Here's how the part is built. I have some questions about the finished solid (model axes, mm). A direction names the side the tool comes from. Give positions to 0.01 mm unless a question says otherwise; leave off trailing zeros. Order: outer loops, then holes, each group sorted by start corner. A loop starts at its lowest first (then second) coordinate and runs counter-clockwise, first axis right, second up. Notation, with made-up numbers: (-14.75, 74.25) -> (0.25, 74.25) arc R8 ccw to (0.25, 84.25) -> close; hole circle Ø1 at (35.5, 69.5). An arc over 180 degrees is marked (long way). Write each question's results on one line, items separated by ' | '. Start each with the question number.
Q1. Thinking about a two-plate mould opening in Y: for faces 1 (the face through (2, -12, 0)), 2 (the face through (2, 18.918, 5)), 3 (the face through (34.04, -44.075, 0.986)), which applies, pulls with the +Y half, pulls with the -Y half, needs draft (parallel to the pull), parting line crosses it, or undercut?
Q2. Imagine slicing it at A-A, the plane z = 5. Please give me the cut outline in (x, y), then the cut area to 3 significant figures.
Q3. I need wall thicknesses on line 1 along Y through (x, z) = (26.5, 5); line 2 along X through (y, z) = (-32.5, 8.5); line 3 along Z through (x, y) = (-9.5, -15). Which ranges of each line are inside material? Lowest first, please. Write a range as [from, to].
Q4. Imagine slicing it at C-C, the plane x = -18. Please give me the cut outline in (y, z), then the cut area to 3 significant figures.
Q5. For faces 4 (the face through (31.087, 17.207, 5.451)), 5 (the face through (33.91, 7.35, 5.45)), 6 (the face through (32.61, -42.676, 5.451)), which set-ups out of +Z, -Z, +X, -X, +Y, -Y let a thin tool reach every point of the face, with its end or its side?
Q6. Imagine slicing it at B-B, the plane y = 3. Please give me the cut outline in (x, z), then the cut area to 3 significant figures.
Q7. I'm going to push flat-ended pins straight in: pin 1 (2 mm diameter, centred on y = -2.5, z = 4, fed in from +X); pin 2 (6 mm diameter, centred on x = -3.5, y = -10, fed in from +Z); pin 3 (1.8 mm diameter, centred on y = 5.92, z = 5, fed in from -X). Where does each tip first touch, or does it pass through?
```python
from build123d import *

# Parameters (mm, degrees)
EXTRUDE_1_DEPTH     = 2
EXTRUDE_2_DEPTH     = 7
SHELL_1_T           = -2
SKETCH_3_R          = 1.5
CUT_EXTRUDE_1_DEPTH = 7
SKETCH_4_R          = 1.5
CUT_EXTRUDE_2_DEPTH = 7


with BuildPart() as part:
    # 草图1 → 凸台-拉伸1 (new body)
    with BuildSketch(Plane.XY):
        with BuildLine():
            Line((-23.108505897, 22.918009168), (26.891494103, 22.918009168))
            ThreePointArc((26.891494103, 22.918009168), (33.962561915, 19.989076979), (36.891494103, 12.918009168))
            Line((36.891494103, 12.918009168), (36.891494103, -37.081990832))
            ThreePointArc((36.891494103, -37.081990832), (33.962561915, -44.153058644), (26.891494103, -47.081990832))
            Line((26.891494103, -47.081990832), (-23.108505897, -47.081990832))
            ThreePointArc((-23.108505897, -47.081990832), (-30.179573709, -44.153058644), (-33.108505897, -37.081990832))
            Line((-33.108505897, -37.081990832), (-33.108505897, 12.918009168))
            ThreePointArc((-33.108505897, 12.918009168), (-30.179573709, 19.989076979), (-23.108505897, 22.918009168))
        make_face()
    extrude(amount=EXTRUDE_1_DEPTH)

    # 草图2 → 凸台-拉伸2 (add)
    with BuildSketch(Plane.XY.offset(2)):
        with BuildLine():
            Line((-23.108505897, 20.918009168), (26.891494103, 20.918009168))
            ThreePointArc((26.891494103, 20.918009168), (32.548348353, 18.574863417), (34.891494103, 12.918009168))
            Line((34.891494103, 12.918009168), (34.891494103, -37.081990832))
            ThreePointArc((34.891494103, -37.081990832), (32.548348353, -42.738845082), (26.891494103, -45.081990832))
            Line((26.891494103, -45.081990832), (-23.108505897, -45.081990832))
            ThreePointArc((-23.108505897, -45.081990832), (-28.765360146, -42.738845082), (-31.108505897, -37.081990832))
            Line((-31.108505897, -37.081990832), (-31.108505897, 12.918009168))
            ThreePointArc((-31.108505897, 12.918009168), (-28.765360146, 18.574863417), (-23.108505897, 20.918009168))
        make_face()
    extrude(amount=EXTRUDE_2_DEPTH)

    # 抽壳1
    shell_1_openings = [part.faces().sort_by_distance(p)[0] for p in [
        (1.891494103, -12.081990832, 9),
    ]]
    offset(amount=SHELL_1_T, openings=shell_1_openings, kind=Kind.INTERSECTION)

    # 草图3 → 切除-拉伸1 (cut)
    with BuildSketch(Plane.ZY.offset(31.108505897)):
        with Locations(Location((5, -30.081990832, 0), (0, 0, 270))):
            Circle(SKETCH_3_R)
    extrude(amount=-CUT_EXTRUDE_1_DEPTH, mode=Mode.SUBTRACT)

    # 草图4 → 切除-拉伸2 (cut)
    with BuildSketch(Plane(origin=(34.891494103, 0, 0), x_dir=(0, 0, -1), z_dir=(1, 0, 0))):
        with Locations(Location((-5, 5.918009168, 0), (0, 0, 90))):
            Circle(SKETCH_4_R)
    extrude(amount=-CUT_EXTRUDE_2_DEPTH, mode=Mode.SUBTRACT)


solid = part.part
```
Geometry check:
1) face 1: needs draft | face 2: undercut | face 3: pulls with the -Y half
2) outline: (-31.11, -37.08) arc R8 ccw to (-23.11, -45.08) -> (26.89, -45.08) arc R8 ccw to (34.89, -37.08) -> (34.89, 4.42) -> (32.89, 4.42) -> (32.89, -37.08) arc R6 cw to (26.89, -43.08) -> (-23.11, -43.08) arc R6 cw to (-29.11, -37.08) -> (-29.11, -31.58) -> (-31.11, -31.58) -> close; (-31.11, -28.58) -> (-29.11, -28.58) -> (-29.11, 12.92) arc R6 cw to (-23.11, 18.92) -> (26.89, 18.92) arc R6 cw to (32.89, 12.92) -> (32.89, 7.42) -> (34.89, 7.42) -> (34.89, 12.92) arc R8 ccw to (26.89, 20.92) -> (-23.11, 20.92) arc R8 ccw to (-31.11, 12.92) -> close | area: 476 mm²
3) line 1: [-45.08, -43.08], [18.92, 20.92] | line 2: [-31.11, -29.11], [32.89, 34.89] | line 3: [0, 2]
4) outline: (-47.08, 0) -> (22.92, 0) -> (22.92, 2) -> (20.92, 2) -> (20.92, 9) -> (18.92, 9) -> (18.92, 2) -> (-43.08, 2) -> (-43.08, 9) -> (-45.08, 9) -> (-45.08, 2) -> (-47.08, 2) -> close | area: 168 mm²
5) face 4: +Z | face 5: +X | face 6: +Z, +X, -Y
6) outline: (-33.11, 0) -> (36.89, 0) -> (36.89, 2) -> (34.89, 2) -> (34.89, 9) -> (32.89, 9) -> (32.89, 2) -> (-29.11, 2) -> (-29.11, 9) -> (-31.11, 9) -> (-31.11, 2) -> (-33.11, 2) -> close | area: 168 mm²
7) pin 1: x = 34.89 | pin 2: z = 2 | pin 3: x = -31.11
